from build123d import *

# Parameters (mm, degrees)
SKETCH_1_R          = 2.1
EXTRUDE_1_DEPTH     = 650
FILLET_1_R          = 1
SKETCH_4_W          = 20.710237558
SKETCH_4_H          = 20.933829866
CUT_EXTRUDE_1_DEPTH = 438


with BuildPart() as part:
    # 草图1 → 凸台-拉伸1 (new body)
    with BuildSketch(Plane(origin=(0, 0, 0), x_dir=(1, 0, 0), z_dir=(0, 1, 0))):
        Polygon((10, 10), (3, 10), (3, 8), (6, 8), (2, 4), (-2, 4), (-6, 8), (-3, 8), (-3, 10), (-10, 10), (-10, 3), (-8, 3), (-8, 6), (-4, 2), (-4, -2), (-8, -6), (-8, -3), (-10, -3), (-10, -10), (-3, -10), (-3, -8), (-6, -8), (-2, -4), (2, -4), (6, -8), (3, -8), (3, -10), (10, -10), (10, -3), (8, -3), (8, -6), (4, -2), (4, 2), (8, 6), (8, 3), (10, 3), align=None)
        with Locations(Location((0, 0, 0), (0, 0, 270))):
            Circle(SKETCH_1_R, mode=Mode.SUBTRACT)
    extrude(amount=EXTRUDE_1_DEPTH)

    # 圆角1
    fillet_1_edges = [part.edges().sort_by_distance(p)[0] for p in [
        (10, 325, 10),
        (-10, 325, 10),
        (-10, 325, -10),
        (10, 325, -10),
    ]]
    fillet(fillet_1_edges, radius=FILLET_1_R)

    # 草图4 → 切除-拉伸1 (cut)
    with BuildSketch(Plane(origin=(0, 650, 0), x_dir=(1, 0, 0), z_dir=(0, 1, 0))):
        Rectangle(SKETCH_4_W, SKETCH_4_H)
    extrude(amount=-CUT_EXTRUDE_1_DEPTH, mode=Mode.SUBTRACT)


solid = part.part
Here's how the part is built. I have some questions about the finished solid (model axes, mm). Round coordinates to 2 decimals unless told otherwise and drop trailing zeros. Order: outer loops, then holes, each group sorted by start corner. A loop starts at its lowest first (then second) coordinate and runs counter-clockwise, first axis right, second up. Notation, with made-up numbers: (86, 61) -> (104, 61) arc R12 ccw to (104, 78) -> close; hole circle Ø8 at (-10.5, 57.25). An arc over 180 degrees is marked (long way). Return JSON: item names as keys, results as strings.
Q1. I need wall thicknesses on line 1 along Z through (x, y) = (9, 31); line 2 along Z through (x, y) = (0, 86); line 3 along X through (y, z) = (124, 0.25). Which ranges of each line are inside material? Lowest first, please. Write a range as from..to.
Filled sheet:
{"line 1": "z = -10..-3, 3..10", "line 2": "z = -4..-2.1, 2.1..4", "line 3": "x = -4..-2.09, 2.09..4"}
Q2. If we section it at A-A on x = 0: List the corners of the cut face in (y, z) for me, plus the area to 3 significant figures.
Filled sheet:
{"outline": "(0, -4) -> (212, -4) -> (212, -2.1) -> (0, -2.1) -> close; (0, 2.1) -> (212, 2.1) -> (212, 4) -> (0, 4) -> close", "area": "806 mm^2"}
Q3. For pin 1 Ø3 at (x, y) = (0, 120.5) entering from -Z; pin 2 Ø1.2 at (y, z) = (70, -1) entering from +X, each with a flat end and sliding along its axis, tell me the tip position at first contact or that it passes through.
Filled sheet:
{"pin 1": "stops at z = -4", "pin 2": "stops at x = 4"}
Q4. If we section it at B-B on z = 0: List the corners of the cut face in (x, y) for me.
Filled sheet:
{"outline": "(-4, 0) -> (-2.1, 0) -> (-2.1, 212) -> (-4, 212) -> close; (2.1, 0) -> (4, 0) -> (4, 212) -> (2.1, 212) -> close"}
Q5. If we mould it in two halves opening along Z, with no side actions, what happens to faces 1 (the flat face through (6, 105, -4)), 2 (the flat face through (4, 105, 6)), 3 (the flat face through (10, 105, -6)), 4 (the flat face through (0, 105, 4))? For each: released by +Z, released by -Z, zero draft, split by the parting line, or undercut.
Filled sheet:
{"face 1": "undercut", "face 2": "undercut", "face 3": "zero draft", "face 4": "released by +Z"}
